For this review, take the finished solid that the model builds, in its own axes (mm). A direction names the side the tool comes from. Round coordinates to 2 decimals unless told otherwise and drop trailing zeros. Order: outer loops, then holes, each group sorted by start corner. A loop starts at its lowest first (then second) coordinate and runs counter-clockwise, first axis right, second up.
from build123d import *

# Parameters (mm, degrees)
F1_DEPTH = 9


with BuildPart() as f1:
    # F0 (on Top) → F1 (new body)
    with BuildSketch(Plane.XY):
        with BuildLine():
            Line((-4.188961, -2.4), (4.5, -2.4))
            Line((4.5, -2.4), (3.172631, -0.811589))
            ThreePointArc((3.172631, -0.811589), (3.065694, -0.729275), (2.933958, -0.7))
            Line((2.933958, -0.7), (2.6, -0.7))
            Line((2.6, -0.7), (2.6, -1.5))
            Line((2.6, -1.5), (-2.588961, -1.5))
            ThreePointArc((-2.588961, -1.5), (-2.808899, -1.408899), (-2.9, -1.188961))
            Line((-2.9, -1.188961), (-2.9, 1.188961))
            ThreePointArc((-2.9, 1.188961), (-2.808899, 1.408899), (-2.588961, 1.5))
            Line((-2.588961, 1.5), (2.6, 1.5))
            Line((2.6, 1.5), (2.6, 0.7))
            Line((2.6, 0.7), (2.933958, 0.7))
            ThreePointArc((2.933958, 0.7), (3.065694, 0.729275), (3.172631, 0.811589))
            Line((3.172631, 0.811589), (4.5, 2.4))
            Line((4.5, 2.4), (-4.188961, 2.4))
            ThreePointArc((-4.188961, 2.4), (-4.408899, 2.308899), (-4.5, 2.088961))
            Line((-4.5, 2.088961), (-4.5, -2.088961))
            ThreePointArc((-4.5, -2.088961), (-4.408899, -2.308899), (-4.188961, -2.4))
        make_face()
    extrude(amount=F1_DEPTH)


solid = f1.part
(1) Wall thickness on L1, parallel to Y at x = -0.75, z = 6.25; L2, parallel to X at y = 1.15, z = 8.5; L3, parallel to X at y = 1.35, z = 8.25: over which ranges is each line inside the solid? List them lowest first.
(2) Add section D-D on y = 0.05. Give the boundary of the cut face in (x, z), plus the area to 3 significant figures.
(3) Tool access review of faces 1 (the face through (-2.9, 0, 4)), 2 (the face through (3.827, 1.595, 4.437)), 3 (the face through (-1, 2, 0)): name each direction out of +Z, -Z, +X, -X, +Y, -Y from which nothing blocks a thin tool from reaching the whole face with its end or side.
(4) Draft analysis for pull direction X (two halves, no side actions). For faces 4 (the face through (0, -2.4, 4)), 5 (the face through (0, 1.5, 4)), 6 (the face through (-4.5, 0, 4)), state which applies: pulls with the +X half, pulls with the -X half, needs draft (parallel to the pull), parting line crosses it, or undercut.
(5) Add section B-B on z = 6. Give the boundary of the cut face in (x, y), plus the area to 3 significant figures.
(6) Add section A-A on x = -1.75. Give the boundary of the cut face in (y, z).
(7) Clearance check with a flat-ended pin moving along its axis: P1, Ø1.9, axis at y = 0.5, z = 4, coming from the +X side. State where the tip first meets the part, or that it passes through.
(8) Add section C-C on x = 2.75. Give the boundary of the cut face in (y, z), plus the area to 3 significant figures.
Here are the results:
1. L1: y = -2.4 to -1.5, 1.5 to 2.4
1. L2: x = -4.5 to -2.9, 2.6 to 3.46
1. L3: x = -4.5 to -2.86, 2.6 to 3.62
2. outline: (-4.5, 0) - (-2.9, 0) - (-2.9, 9) - (-4.5, 9) - close
2. area: 14.4 mm2
3. face 1: +Z, -Z
3. face 2: +Z, -Z, +X
3. face 3: -Z, +X, -X, +Y, -Y
4. face 4: needs draft
4. face 5: undercut
4. face 6: pulls with the -X half
5. outline: (-4.5, -2.09) arc R0.31 ccw to (-4.19, -2.4) - (4.5, -2.4) - (3.17, -0.81) arc R0.31 ccw to (2.93, -0.7) - (2.6, -0.7) - (2.6, -1.5) - (-2.59, -1.5) arc R0.31 cw to (-2.9, -1.19) - (-2.9, 1.19) arc R0.31 cw to (-2.59, 1.5) - (2.6, 1.5) - (2.6, 0.7) - (2.93, 0.7) arc R0.31 ccw to (3.17, 0.81) - (4.5, 2.4) - (-4.19, 2.4) arc R0.31 ccw to (-4.5, 2.09) - close
5. area: 21.6 mm2
6. outline: (-2.4, 0) - (-1.5, 0) - (-1.5, 9) - (-2.4, 9) - close; (1.5, 0) - (2.4, 0) - (2.4, 9) - (1.5, 9) - close
7. P1: stops at x = 3.71
8. outline: (-2.4, 0) - (-0.7, 0) - (-0.7, 9) - (-2.4, 9) - close; (0.7, 0) - (2.4, 0) - (2.4, 9) - (0.7, 9) - close
8. area: 30.6 mm2
